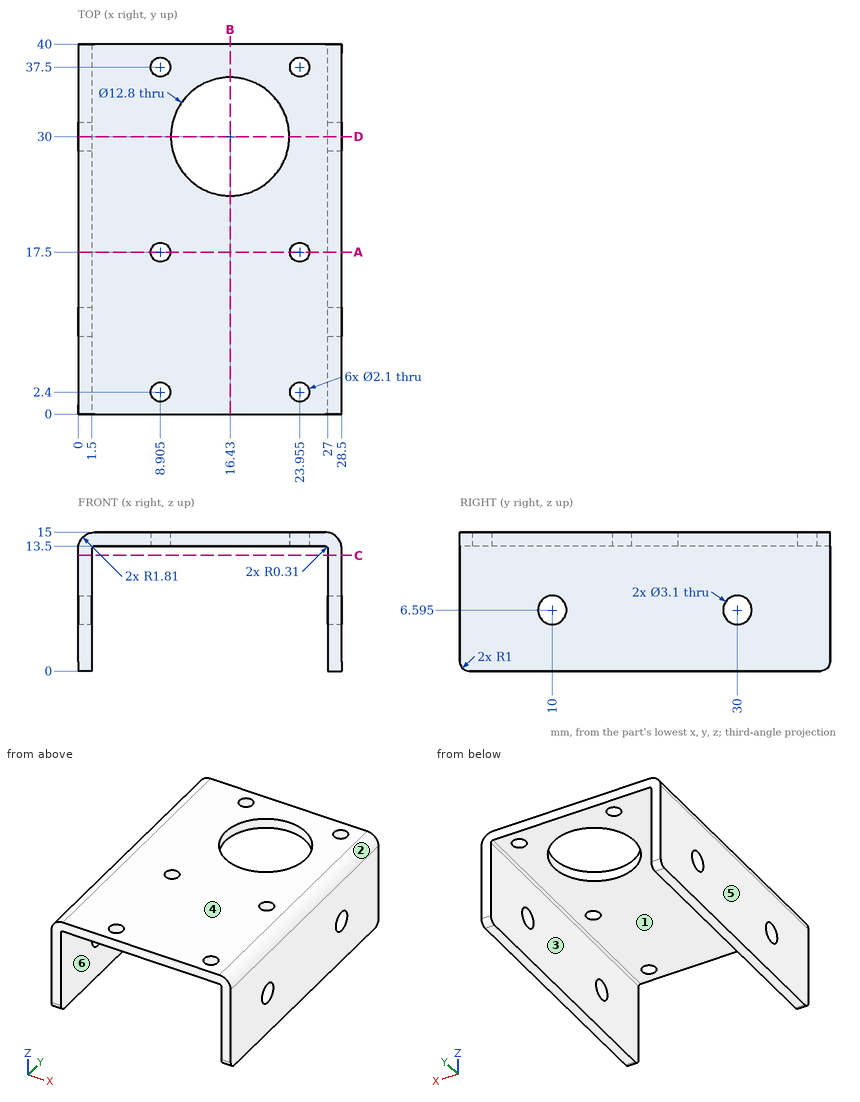
Geometry check sheet. Reference: drawing and pictorial views, mm from the part's lowest x, y, z. A direction names the side the tool comes from. Give positions to 0.01 mm unless a question says otherwise; leave off trailing zeros. Write each loop counter-clockwise with the first axis right and the second up, starting at its lowest first coordinate (ties: lowest second). Pieces come first, ordered by that corner, then holes. Notation, with made-up numbers: (78, 48.5) - (111, 48.5) arc R19 ccw to (111, 64.5) - close; hole circle Ø10 at (45, 21.5). An arc over 180 degrees is marked (long way). Put each result on its own line as item: value.
Q1. Section check D-D on y = 30. Record the cut outline in (x, z) (3 decimals).
Result:
outline: (0, 0) - (1.5, 0) - (1.5, 5.045) - (0, 5.045) - close; (0, 8.145) - (1.5, 8.145) - (1.5, 13.19) arc R0.31 cw to (1.81, 13.5) - (10.03, 13.5) - (10.03, 15) - (1.81, 15) arc R1.81 ccw to (0, 13.19) - close; (22.83, 13.5) - (26.69, 13.5) arc R0.31 cw to (27, 13.19) - (27, 8.145) - (28.5, 8.145) - (28.5, 13.19) arc R1.81 ccw to (26.69, 15) - (22.83, 15) - close; (27, 0) - (28.5, 0) - (28.5, 5.045) - (27, 5.045) - close
Q2. Depth check by flat-ended pin: P1, Ø6, axis at x = 7, y = 13.5, coming from the -Z side. Enter the tip coordinate at first touch or a pass-through.
Result:
P1: z = 13.5
Q3. Scan lines: probe 1 along X at (y, z) = (6.5, 9.75); probe 2 along Z at (x, y) = (5, 11); probe 3 along X at (y, z) = (2.4, 14.2) (3 decimals). Record each from-to range of solid material in increasing order. Write a range as from..to.
Result:
probe 1: 0..1.5, 27..28.5
probe 2: 13.5..15
probe 3: 0.308..7.855, 9.955..22.905, 25.005..28.192
Q4. Set-up check for the marked faces 5 and 6: record each of +Z, -Z, +X, -X, +Y, -Y from which the full face is reachable in a straight line by a thin tool's end or side.
Result:
face 5: +Z, -Z, -X, +Y, -Y
face 6: -Z, +Y, -Y
Q5. Mould release check, pull along X, two halves, no side actions. Record for the marked faces 1, 2, 3 and 4: released by +X, released by -X, zero draft, split by the parting line, or undercut.
Result:
face 1: undercut
face 2: released by +X
face 3: undercut
face 4: zero draft
Q6. Section check C-C on z = 12.5. Record the cut outline in (x, y).
Result:
outline: (0, 0) - (1.5, 0) - (1.5, 40) - (0, 40) - close; (27, 0) - (28.5, 0) - (28.5, 40) - (27, 40) - close
Q7. Section check A-A on y = 17.5. Record the cut outline in (x, z) (3 decimals).
Result:
outline: (0, 0) - (1.5, 0) - (1.5, 13.19) arc R0.31 cw to (1.81, 13.5) - (7.855, 13.5) - (7.855, 15) - (1.81, 15) arc R1.81 ccw to (0, 13.19) - close; (9.955, 13.5) - (22.905, 13.5) - (22.905, 15) - (9.955, 15) - close; (25.005, 13.5) - (26.69, 13.5) arc R0.31 cw to (27, 13.19) - (27, 0) - (28.5, 0) - (28.5, 13.19) arc R1.81 ccw to (26.69, 15) - (25.005, 15) - close
Q8. Section check B-B on x = 16.43. Record the cut outline in (y, z), and give its area (3 significant figures).
Result:
outline: (0, 13.5) - (23.6, 13.5) - (23.6, 15) - (0, 15) - close; (36.4, 13.5) - (40, 13.5) - (40, 15) - (36.4, 15) - close
area: 40.8 mm2
